```python
from build123d import *

# Parameters (mm, degrees)
BOSS_EXTRUDE1_DEPTH             = 26
SKETCH4_W                       = 32.5
SKETCH4_H                       = 67.5
CUT_EXTRUDE1_DEPTH              = 20
SKETCH5_R                       = 2.525
CUT_EXTRUDE2_DEPTH              = 557.471248134
SKETCH6_W                       = 8
SKETCH6_H                       = 67.5
BOSS_EXTRUDE2_DEPTH             = 20
FILLET3_R                       = 4
SKETCH9_R                       = 3.25
CUT_EXTRUDE3_DEPTH              = 5
M3X0_5_TAPPED_HOLE1_D           = 2.5
M3X0_5_TAPPED_HOLE1_DEPTH       = 10
M3X0_5_TAPPED_HOLE1_CSINK_D     = 3.05
M3X0_5_TAPPED_HOLE1_CSINK_ANGLE = 90
M3X0_5_TAPPED_HOLE1_TIP         = 0.751075774


with BuildPart() as part:
    # Sketch3 → Boss-Extrude1 (new body)
    with BuildSketch(Plane.XY):
        with BuildLine():
            Line((516, 38.526197832), (504.607604335, 38.526197832))
            ThreePointArc((504.607604335, 38.526197832), (501.779177211, 37.354624957), (500.607604335, 34.526197832))
            Line((500.607604335, 34.526197832), (500.607604335, 24))
            Line((500.607604335, 24), (500.607604335, 0))
            Line((500.607604335, 0), (516, 0))
            Line((516, 0), (552, 0))
            Line((552, 0), (552, 38.526197832))
            Line((552, 38.526197832), (552, 67.5))
            Line((552, 67.5), (520, 67.5))
            Line((520, 67.5), (520, 42.526197832))
            ThreePointArc((520, 42.526197832), (518.828427125, 39.697770708), (516, 38.526197832))
        make_face()
    extrude(amount=BOSS_EXTRUDE1_DEPTH)

    # Sketch4 → Cut-Extrude1 (cut)
    with BuildSketch(Plane(origin=(0, 0, 0), x_dir=(-1, 0, 0), z_dir=(0, 0, -1))):
        with Locations((-516.857604335, 33.75)):
            Rectangle(SKETCH4_W, SKETCH4_H)
    extrude(amount=-CUT_EXTRUDE1_DEPTH, mode=Mode.SUBTRACT)

    # Sketch5 → Cut-Extrude2 (cut, through all)
    with BuildSketch(Plane(origin=(0, 0, 20), x_dir=(-1, 0, 0), z_dir=(0, 0, -1))):
        with Locations((-510.767604335, 28.366197832)):
            Circle(SKETCH5_R)
        with Locations((-510.767604335, 15.636197832)):
            Circle(SKETCH5_R)
    extrude(amount=-CUT_EXTRUDE2_DEPTH, mode=Mode.SUBTRACT)

    # Sketch6 → Boss-Extrude2 (add)
    with BuildSketch(Plane(origin=(0, 0, 20), x_dir=(-1, 0, 0), z_dir=(0, 0, -1))):
        with Locations((-524, 33.75)):
            Rectangle(SKETCH6_W, SKETCH6_H)
    extrude(amount=BOSS_EXTRUDE2_DEPTH)

    # Fillet3
    fillet3_edges = [part.edges().sort_by_distance(p)[0] for p in [
        (520, 67.5, 13),
        (552, 67.5, 13),
        (552, 0, 13),
        (500.607604335, 0, 23),
        (520, 0, 10),
    ]]
    fillet(fillet3_edges, radius=FILLET3_R)

    # Sketch9 → Cut-Extrude3 (cut)
    with BuildSketch(Plane(origin=(0, 0, 0), x_dir=(-1, 0, 0), z_dir=(0, 0, -1))):
        with Locations((-523.5, 5)):
            Circle(SKETCH9_R)
        with Locations((-548.5, 5)):
            Circle(SKETCH9_R)
    extrude(amount=-CUT_EXTRUDE3_DEPTH, mode=Mode.SUBTRACT)

    # M3x0.5 Tapped Hole1
    with Locations(Plane(origin=(0, 0, 0), x_dir=(-1, 0, 0), z_dir=(0, 0, -1))):
        with Locations((-523.5, 57.5), (-548.5, 57.5), (-548.5, 22.5), (-523.5, 22.5)):
            CounterSinkHole(M3X0_5_TAPPED_HOLE1_D / 2, M3X0_5_TAPPED_HOLE1_CSINK_D / 2, depth=M3X0_5_TAPPED_HOLE1_DEPTH, counter_sink_angle=M3X0_5_TAPPED_HOLE1_CSINK_ANGLE)
            with Locations((0, 0, -(M3X0_5_TAPPED_HOLE1_DEPTH + M3X0_5_TAPPED_HOLE1_TIP / 2))):  # 118° drill point
                Cone(0, M3X0_5_TAPPED_HOLE1_D / 2, M3X0_5_TAPPED_HOLE1_TIP, mode=Mode.SUBTRACT)


solid = part.part
```
Geometry check sheet. Reference: the model listing, model coordinates, mm. A direction names the side the tool comes from. Coordinates: 2 decimals unless noted, no trailing zeros. Write each loop counter-clockwise with the first axis right and the second up, starting at its lowest first coordinate (ties: lowest second). Pieces come first, ordered by that corner, then holes. Notation, with made-up numbers: M 57,58 L 115,58 A19 cw 115,62 Z; hole C 14.5,40 d6. An arc over 180 degrees is marked long. Answer as a JSON object with one key per item and string values.
1. Section check A-A, the plane z = 3. Enter the section's corners in (x, y).
Answers below:
{"outline": "M 520,4 A4 ccw 524,0 L 528,0 L 528,67.5 L 524,67.5 A4 ccw 520,63.5 Z; M 533.11,0 L 548,0 A4 ccw 552,4 L 552,63.5 A4 ccw 548,67.5 L 533.11,67.5 Z; hole C 523.5,5 d6.5; hole C 523.5,22.5 d2.5; hole C 523.5,57.5 d2.5; hole C 548.5,5 d6.5; hole C 548.5,22.5 d2.5; hole C 548.5,57.5 d2.5"}
2. Draft check along X on faces 4 (the flat face through (539, 67.5, 13)), 5 (the conical face through (548.3, 22.42, 10.62)), 6 (the cylindrical face through (521.141, 66.297, 13.182)). Enter one of: released by +X, released by -X, zero draft, split by the parting line, or undercut.
Answers below:
{"face 4": "zero draft", "face 5": "undercut", "face 6": "released by -X"}
3. Section check C-C, the plane z = 14.5. Enter the section's corners in (x, y).
Answers below:
{"outline": "M 520,4 A4 ccw 524,0 L 528,0 L 528,67.5 L 524,67.5 A4 ccw 520,63.5 Z; M 533.11,0 L 548,0 A4 ccw 552,4 L 552,63.5 A4 ccw 548,67.5 L 533.11,67.5 Z"}
4. Scan lines: L1, parallel to X at y = 57.5, z = 4.75; L2, parallel to X at y = 25.5, z = 5.75; L3, parallel to Y at x = 523.5, z = 2.2. Record each from-to range of solid material in increasing order.
Answers below:
{"L1": "x = 520 to 522.25, 524.75 to 528, 533.11 to 547.25, 549.75 to 552", "L2": "x = 520 to 528, 533.11 to 552", "L3": "y = 0.03 to 1.75, 8.25 to 21.25, 23.75 to 56.25, 58.75 to 67.47"}
5. Go/stop test with flat-tipped pins: pin 1 Ø5 at (x, z) = (520.5, 14) entering from -Y; pin 2 Ø2 at (x, y) = (548.5, 57.5) entering from -Z; pin 3 Ø1.8 at (x, z) = (512, 23) entering from +Y. Record where each tip stops, or that it passes through.
Answers below:
{"pin 1": "stops at y = 0.13", "pin 2": "stops at z = 10.15", "pin 3": "stops at y = 38.53"}
6. Section check B-B, the plane y = 19.5. Enter the section's corners in (x, z).
Answers below:
{"outline": "M 500.61,20 L 520,20 L 520,0 L 528,0 L 528,20 L 533.11,20 L 533.11,0 L 552,0 L 552,26 L 500.61,26 Z"}
7. Section check D-D, the plane y = 5. Enter the section's corners in (x, z), plus the area to 3 significant figures.
Answers below:
{"outline": "M 500.61,20 L 520,20 L 520,0 L 520.25,0 L 520.25,5 L 526.75,5 L 526.75,0 L 528,0 L 528,20 L 533.11,20 L 533.11,0 L 545.25,0 L 545.25,5 L 551.75,5 L 551.75,0 L 552,0 L 552,26 L 500.61,26 Z", "area": "781 mm²"}
8. Tool access check on faces 1 (the flat face through (533.108, 33, 10)), 2 (the cylindrical face through (513.29, 28.48, 22.96)), 3 (the cylindrical face through (547.25, 22.55, 5.21)). Record the directions out of +Z, -Z, +X, -X, +Y, -Y that give a thin tool (end or side, any length) a straight path to the whole face; none if there is none.
Answers below:
{"face 1": "-Z, +Y, -Y", "face 2": "+Z, -Z", "face 3": "-Z"}
